```python
from build123d import *

# Parameters (mm, degrees)
SKETCH1_W             = 75
SKETCH1_H             = 120
SKETCH1_R             = 4
BOSS_EXTRUDE1_DEPTH   = 18
F_1_0MM_DOWEL_HOLE1_D = 12


with BuildPart() as part:
    # Sketch1 → Boss-Extrude1 (new body)
    with BuildSketch(Plane.XY):
        Rectangle(SKETCH1_W, SKETCH1_H)
        with Locations((8.5, 33)):
            Circle(SKETCH1_R, mode=Mode.SUBTRACT)
        with Locations((8.5, -33)):
            Circle(SKETCH1_R, mode=Mode.SUBTRACT)
    extrude(amount=BOSS_EXTRUDE1_DEPTH)

    # Ø1.0mm Dowel Hole1 (through all)
    with Locations(Plane(origin=(0, 0, 0), x_dir=(-1, 0, 0), z_dir=(0, 0, -1))):
        with Locations((-0.5, 0)):
            Hole(F_1_0MM_DOWEL_HOLE1_D / 2)


solid = part.part
```
Verification items for the finished model (mm, model axes). Round coordinates to 2 decimals unless told otherwise and drop trailing zeros. Order: outer loops, then holes, each group sorted by start corner. A loop starts at its lowest first (then second) coordinate and runs counter-clockwise, first axis right, second up.
1) Draft check along Y on faces 1 (the flat face through (-1, 60, 9)), 2 (the flat face through (-37.5, -1, 9)), 3 (the cylindrical face through (7.979, 36.966, 8.874)). Enter one of: +Y half, -Y half, draft (parallel to the pull), parting line (faces both ways), or undercut.
Geometry says:
face 1: +Y half
face 2: draft
face 3: undercut
2) Cross-section at C-C, the plane z = 3. Record the cut outline in (x, y).
Geometry says:
outline: (-37.5, -60) - (37.5, -60) - (37.5, 60) - (-37.5, 60) - close; hole circle Ø12 at (0.5, 0); hole circle Ø8 at (8.5, -33); hole circle Ø8 at (8.5, 33)
3) Cross-section at B-B, the plane x = 8.5. Record the cut outline in (y, z), plus the area to 3 significant figures.
Geometry says:
outline: (-60, 0) - (-37, 0) - (-37, 18) - (-60, 18) - close; (-29, 0) - (29, 0) - (29, 18) - (-29, 18) - close; (37, 0) - (60, 0) - (60, 18) - (37, 18) - close
area: 1,870 mm2
4) Material ranges on line 1 (Y direction, x = 8.5, z = 6); line 2 (Y direction, x = 0.5, z = 10.75); line 3 (X direction, y = 31, z = 16.25), recorded low to high.
Geometry says:
line 1: y = -60 to -37, -29 to 29, 37 to 60
line 2: y = -60 to -6, 6 to 60
line 3: x = -37.5 to 5.04, 11.96 to 37.5
5) Cross-section at A-A, the plane y = 0. Record the cut outline in (x, z).
Geometry says:
outline: (-37.5, 0) - (-5.5, 0) - (-5.5, 18) - (-37.5, 18) - close; (6.5, 0) - (37.5, 0) - (37.5, 18) - (6.5, 18) - close
6) Cross-section at D-D, the plane y = -33. Record the cut outline in (x, z), plus the area to 3 significant figures.
Geometry says:
outline: (-37.5, 0) - (4.5, 0) - (4.5, 18) - (-37.5, 18) - close; (12.5, 0) - (37.5, 0) - (37.5, 18) - (12.5, 18) - close
area: 1,210 mm2
